```python
from build123d import *

# Parameters (mm, degrees)
F1_DEPTH  = 74.422
F3_DEPTH  = 25.4
F5_DEPTH  = 25.4
F7_DEPTH  = 3.81
F9_DEPTH  = 1.778
F11_DEPTH = 1.778


with BuildPart() as f1:
    # F0 (on Top) → F1 (new body)
    with BuildSketch(Plane.XY):
        Polygon((13.9353908598, 24.9320268631), (-12.7978082746, 24.9320268631), (0, -34.9806770682), align=None)
    extrude(amount=F1_DEPTH)

    # F2 (on face) → F3 (cut)
    with BuildSketch(Plane(origin=(7.718740982, -1.7953399775, 0), x_dir=(0.226547485, 0.9740001217, 0), z_dir=(0.9740001217, -0.226547485, 0))):
        Polygon((20.695079118, 52.2201247513), (-34.0711837213, 74.422), (-34.0711837213, 39.8090481758), align=None)
    extrude(amount=-F3_DEPTH, mode=Mode.SUBTRACT)

    # F4 (on face) → F5 (cut)
    with BuildSketch(Plane(origin=(-7.1460755316, -1.5264559696, 0), x_dir=(0.2088949953, -0.9779380762, 0), z_dir=(-0.9779380762, -0.2088949953, 0))):
        Polygon((34.2089360376, 0), (34.2089360376, 39.8090481758), (-23.0083428323, 20.9681969136), align=None)
    extrude(amount=-F5_DEPTH, mode=Mode.SUBTRACT)

    # F6 (on face) → F7 (cut)
    with BuildSketch(Plane(origin=(-7.1460755316, -1.5264559696, 0), x_dir=(0.2088949953, -0.9779380762, 0), z_dir=(-0.9779380762, -0.2088949953, 0))):
        Polygon((14.3255656585, 73.5306164718), (-25.4703722894, 73.2393935323), (-25.4703722894, 53.7560619414), (22.024974227, 71.4815631509), (25.38343653, 72.7349581039), (27.5516982051, 73.5306164718), align=None)
    extrude(amount=-F7_DEPTH, mode=Mode.SUBTRACT)

    # F8 (on face) → F9 (cut)
    with BuildSketch(Plane(origin=(-7.1460755316, -1.5264559696, 0), x_dir=(0.2088949953, -0.9779380762, 0), z_dir=(-0.9779380762, -0.2088949953, 0))):
        Polygon((20.7908283919, 41.430156678), (-25.4458747804, 50.9817264974), (-25.4333440341, 22.6434153364), (-24.5192568436, 22.9174265555), (16.8412234634, 35.3158451617), (31.0665536672, 39.5800992846), align=None)
    extrude(amount=-F9_DEPTH, mode=Mode.SUBTRACT)

    # F10 (on face) → F11 (cut)
    with BuildSketch(Plane(origin=(4.7807632282, 20.554030722, 52.0548786677), x_dir=(0.9963713167, -0.031258558, -0.0791650292), z_dir=(-0.0851128621, -0.3659274261, -0.9267431788))):
        Polygon((5.2179168689, 4.4931433875), (-5.1948507316, 51.9638061523), (-15.6265430034, 0), align=None)
    extrude(amount=-F11_DEPTH, mode=Mode.SUBTRACT)


solid = f1.part
```
CAD build for the part. Positions are in the model's coordinates, mm. A direction names the side the tool comes from. Give positions to 0.01 mm unless a question says otherwise; leave off trailing zeros. Order: outer loops, then holes, each group sorted by start corner. A loop starts at its lowest first (then second) coordinate and runs counter-clockwise, first axis right, second up. Notation, with made-up numbers: M -2.75,45 L 28.25,45 A27 cw 28.25,75 Z; hole C -36,-4 d7. An arc over 180 degrees is marked long. Put each result on its own line as item: value. Start each with the question number.
(1) Saw through at B-B, the plane z = 70. Write the cut outline in (x, y), then the cut area to 3 significant figures.
(2) Mould opens along X. For faces 4 (the flat face through (-9.747, 10.648, 26.012)), 5 (the flat face through (-10.63, 23.774, 63.634)), 6 (the flat face through (9.967, 7.87, 36.69)) say: +X half, -X half, draft (parallel to the pull), parting line (faces both ways), or undercut.
(3) Saw through at D-D, the plane x = 5.5. Write the cut outline in (y, z).
(4) Saw through at C-C, the plane y = -29.5. Write the cut outline in (x, z).
(5) Flat gauge pins, fed straight in: pin 1 Ø2 at (y, z) = (3.5, 33) entering from -X; pin 2 Ø6 at (y, z) = (17, 34.5) entering from +X; pin 3 Ø10 at (y, z) = (-15.5, 39.5) entering from -X; pin 4 Ø4 at (x, y) = (-5, -28.5) entering from -Z. Where does each tip first touch, or does it go through?
(6) Drill centre lines: line 1 along Z through (x, y) = (-1.75, -25); line 2 along Z through (x, y) = (1.5, 12); line 3 along Z through (x, y) = (-6.5, 7). Where is each one in solid material? Low to high.
(7) Saw through at A-A, the plane y = -19.5. Write the cut outline in (x, z), then the cut area to 3 significant figures.
(8) Which spindle directions (+Z, -Z, +X, -X, +Y, -Y) get a long thin tool onto all of the face, cutting with end or side? Do faces 1 (the flat face through (13.395, 23.903, 20.925)), 2 (the flat face through (-6.71, 0.62, 46.14)), 3 (the flat face through (-5.45, -3.33, 63.31)). Say none if no direction does.
Check result:
1. outline: M -12.8,24.93 L -12.47,23.38 L -8.74,24.18 L 0.35,-18.39 L -1.03,-18.68 L 1.57,-19.29 L 0.49,-23.89 L 2.47,-24.36 L 13.94,24.93 Z; M -3.37,-19.18 L -2.52,-23.2 L -1.28,-23.48 L -1.99,-18.89 Z
1. area: 594 mm2
2. face 4: -X half
2. face 5: undercut
2. face 6: +X half
3. outline: M -11.33,0 L 24.93,0 L 24.93,74.42 L -11.33,74.42 L -11.33,64.58 L -2.71,61.18 L -2.7,63.09 L 17.94,54.94 L 17.25,53.29 L 19.97,52.22 L -11.33,45.31 L -11.33,32.57 L 24.7,20.97 L -11.33,8.05 Z
4. outline: M -1.17,0 L 1.27,0 L 1.27,1.87 L -1.17,2.05 Z; M -1.17,37.96 L 1.27,38.13 L 1.27,41.08 L -1.17,40.96 L -1.17,40.02 L 0.65,39.95 L 0.65,38.96 L -1.17,38.84 Z; M -1.17,72.37 L 1.27,72.14 L 1.27,74.42 L -1.17,74.42 Z
5. pin 1: stops at x = -6.62
5. pin 2: stops at x = 12.79
5. pin 3: stops at x = -4.82
5. pin 4: passes through
6. line 1: z = 0 to 3.71, 36.47 to 37.49, 40.84 to 41.92, 70.64 to 72.25, 73.53 to 74.42
6. line 2: z = 0 to 16.72, 24.78 to 50.26, 57.65 to 74.42
6. line 3: z = 0 to 15.54, 25.84 to 48.74, 73.37 to 74.42
7. outline: M -3.31,0 L 3.6,0 L 3.6,5.27 L -3.31,5.8 Z; M -3.31,34.6 L 3.6,35.07 L 3.6,43.41 L -3.31,43.06 L -3.31,41.93 L -1.49,41.85 L -1.49,35.89 L -3.31,35.78 Z; M -3.31,68.61 L -2.13,68.5 L -1.86,70.23 L -3.31,70.12 Z; M -3.31,73.53 L 0.59,73.53 L 0.59,70.42 L -0.89,70.31 L 1.52,70.09 L 1.53,68.17 L 3.6,67.98 L 3.6,74.42 L -3.31,74.42 Z
7. area: 108 mm2
8. face 1: -Y
8. face 2: -X
8. face 3: none
